The model under review builds one solid part; all positions refer to its coordinate system, in mm. A direction names the side the tool comes from. Coordinates: 2 decimals unless noted, no trailing zeros. Order: outer loops, then holes, each group sorted by start corner. A loop starts at its lowest first (then second) coordinate and runs counter-clockwise, first axis right, second up. Notation, with made-up numbers: M 42.5,39 L 100.5,39 A21 cw 100.5,50 Z; hole C 55.5,20.25 d2. An arc over 180 degrees is marked long. Answer in a Markdown table with one row per item.
from build123d import *

# Parameters (mm, degrees)
SKETCH_1_R               = 3.15
SKETCH_1_W               = 77
SKETCH_1_H               = 23
EXTRUDE_1_DEPTH          = 6.6
CUT_EXTRUDE_1_DEPTH      = 46.330012133
CUT_EXTRUDE_1_DEPTH_BACK = 46.330012133
FILLET_1_R               = 3


with BuildPart() as part:
    # 草图1 → 凸台-拉伸1 (new body)
    # profile 1 of 2: a face of its own
    with BuildSketch(Plane(origin=(0, 0, 0), x_dir=(1, 0, 0), z_dir=(0, 1, 0))):
        with BuildLine():
            Line((-5.888001359, 17.775933557), (-11.249562098, 0))
            Line((-11.249562098, 0), (11.249562098, 0))
            Line((11.249562098, 0), (5.888001359, 17.775933557))
            ThreePointArc((5.888001359, 17.775933557), (0, 22.15), (-5.888001359, 17.775933557))
        make_face()
        with Locations(Location((0, 16, 0), (0, 0, 270))):
            Circle(SKETCH_1_R, mode=Mode.SUBTRACT)
    # profile 2 of 2: a face of its own
    with BuildSketch(Plane(origin=(0, 0, 0), x_dir=(1, 0, 0), z_dir=(0, 1, 0))):
        with Locations((0, -11.5)):
            Rectangle(SKETCH_1_W, SKETCH_1_H)
    extrude(amount=EXTRUDE_1_DEPTH)

    # 草图2 → 切除-拉伸1 (cut, two sides: drawn at the far end of the back side and taken through both)
    with BuildSketch(Plane(origin=(0, 0, 0), x_dir=(0, 0, -1), z_dir=(1, 0, 0)).offset(-CUT_EXTRUDE_1_DEPTH_BACK)):
        Polygon((-123.671550114, 2.5), (-23, 2.5), (9.85, 2.5), (9.85, 6.6), (9.85, 107.271550114), (-114.442682903, 265.67095979), (-247.964233016, 160.899409677), align=None)
    extrude(amount=CUT_EXTRUDE_1_DEPTH + CUT_EXTRUDE_1_DEPTH_BACK, mode=Mode.SUBTRACT)

    # 圆角1
    fillet_1_edges = [part.edges().sort_by_distance(p)[0] for p in [
        (0, 6.6, -9.85),
    ]]
    fillet(fillet_1_edges, radius=FILLET_1_R - 0.0001)  # a hair under: the kernel refuses the full size


solid = part.part
(1) Take a section at C-C (z = -16). Write out the cut boundary in (x, y).
Report:
| item | result |
|---|---|
| outline | M -6.42,0 L -3.15,0 L -3.15,6.6 L -6.42,6.6 Z; M 3.15,0 L 6.42,0 L 6.42,6.6 L 3.15,6.6 Z |
(2) Take a section at D-D (x = -21). Write out the cut boundary in (y, z).
Report:
| item | result |
|---|---|
| outline | M 0,0 L 2.5,0 L 2.5,23 L 0,23 Z |
(3) To check wall thickness, follow line 1 (Y direction, x = -26.5, z = 4); line 2 (X direction, y = 3.75, z = -16); line 3 (Z direction, x = 5, y = 2). State the ranges of each line that lie inside material, in increasing order. Write a range as [from, to].
Report:
| item | result |
|---|---|
| line 1 | [0, 2.5] |
| line 2 | [-6.42, -3.15], [3.15, 6.42] |
| line 3 | [-19.58, 23] |
(4) Machinability: for faces 1 (the flat face through (-1, 2.5, 10)), 2 (the flat face through (-25, 1, 0)), 3 (the flat face through (25, 1, 0)), which of the approach directions +Z, -Z, +X, -X, +Y, -Y give a long, thin tool a straight path to every point of the face, cutting with its end or side? Answer none if there is none.
Report:
| item | result |
|---|---|
| face 1 | +Z, +X, -X, +Y |
| face 2 | -Z, -X, +Y, -Y |
| face 3 | -Z, +X, +Y, -Y |
(5) Insertion check: P1, Ø16.5, axis at x = 11, z = 1.5, coming from the +Y side; P2, Ø0.6, axis at x = -4, y = 3, coming from the +Z side; P3, Ø3, axis at x = -31, y = 0.5, coming from the -Z side. Each pin has a flat end and moves straight along its axis. Give the tip position at first contact, or say it passes through.
Report:
| item | result |
|---|---|
| P1 | y = 2.5 |
| P2 | z = -9.85 |
| P3 | z = 0 |
(6) Take a section at B-B (y = 1). Write out the cut boundary in (x, z).
Report:
| item | result |
|---|---|
| outline | M -38.5,0 L -11.25,0 L -5.89,-17.78 A6.15 ccw 5.89,-17.78 L 11.25,0 L 38.5,0 L 38.5,23 L -38.5,23 Z; hole C 0,-16 d6.3 |
